```python
from build123d import *

# Parameters (mm, degrees)
SKETCH_1_W          = 32
SKETCH_1_H          = 86
EXTRUDE_1_DEPTH     = 3
SKETCH_2_W          = 12
SKETCH_2_H          = 3
SKETCH_2_W_2        = 3
CUT_EXTRUDE_1_DEPTH = 4
SKETCH_3_W          = 3
SKETCH_3_H          = 10
CUT_EXTRUDE_2_DEPTH = 4


with BuildPart() as part:
    # 스케치1 → 보스-돌출1 (new body)
    with BuildSketch(Plane.XY):
        with Locations((16, 43)):
            Rectangle(SKETCH_1_W, SKETCH_1_H)
    extrude(amount=EXTRUDE_1_DEPTH)

    # 스케치2 → 컷-돌출1 (cut, through all)
    with BuildSketch(Plane.XY.offset(3)):
        with Locations((16, 84.5)):
            Rectangle(SKETCH_2_W, SKETCH_2_H)
        with Locations((1.5, 84.5)):
            Rectangle(SKETCH_2_W_2, SKETCH_2_H)
        with Locations((30.5, 84.5)):
            Rectangle(SKETCH_2_W_2, SKETCH_2_H)
        with Locations((16, 1.5)):
            Rectangle(SKETCH_2_W, SKETCH_2_H)
        with Locations((1.5, 1.5)):
            Rectangle(SKETCH_2_W_2, SKETCH_2_H)
        with Locations((30.5, 1.5)):
            Rectangle(SKETCH_2_W_2, SKETCH_2_H)
    extrude(amount=-CUT_EXTRUDE_1_DEPTH, mode=Mode.SUBTRACT)

    # 스케치3 → 컷-돌출2 (cut, through all)
    with BuildSketch(Plane.XY.offset(3)):
        with Locations((27.5, 69)):
            Rectangle(SKETCH_3_W, SKETCH_3_H)
        with Locations((4.5, 69)):
            Rectangle(SKETCH_3_W, SKETCH_3_H)
        with Locations((27.5, 17)):
            Rectangle(SKETCH_3_W, SKETCH_3_H)
        with Locations((4.5, 17)):
            Rectangle(SKETCH_3_W, SKETCH_3_H)
    extrude(amount=-CUT_EXTRUDE_2_DEPTH, mode=Mode.SUBTRACT)


solid = part.part
```
Here's how the part is built. I have some questions about the finished solid (model axes, mm). A direction names the side the tool comes from. Give positions to 0.01 mm unless a question says otherwise; leave off trailing zeros. Loops run counter-clockwise (first coordinate to the right, second up) from the corner with the lowest first, then second, coordinate; pieces in that order, holes last. Notation, with made-up numbers: M 70,-10 L 122,-10 A23 ccw 122,10 Z; hole C 11.5,50.25 d4. An arc over 180 degrees is marked long. Put each result on its own line as item: value. Start each with the question number.
(1) I want a section at A-A on x = 4.5. Please give me the cut outline in (y, z).
(2) I want a section at B-B on y = 67.5. Please give me the cut outline in (x, z).
(3) If we mould it in two halves opening along X, with no side actions, what happens to faces 5 (the flat face through (3, 84, 2)), 6 (the flat face through (6, 0, 1)), 7 (the flat face through (22, 1, 2))? For each: +X half, -X half, draft (parallel to the pull), parting line (faces both ways), or undercut.
(4) I need wall thicknesses on line 1 along X through (y, z) = (66.5, 1.2); line 2 along Y through (x, z) = (28.5, 1.5); line 3 along Y through (x, z) = (17, 2.85). Which ranges of each line are inside material? Lowest first, please. Write a range as [from, to].
(5) I want a section at C-C on x = 13.5. Please give me the cut outline in (y, z).
(6) Will this pin go through, and if not, where does the flat tip stop? pin 1 Ø0.9 at (y, z) = (1, 1.5) entering from -X.
(7) For faces 1 (the flat face through (29, 84, 2)), 2 (the flat face through (3, 69, 2)), 3 (the flat face through (16, 83, 2)), 4 (the flat face through (1, 3, 2)), which set-ups out of +Z, -Z, +X, -X, +Y, -Y let a thin tool reach every point of the face, with its end or its side?
(8) I want a section at D-D on z = 0.7. State how many separate pieces and enclosed holes the cut face has, then the cut area to 3 significant figures.
Answer block:
1. outline: M 0,0 L 12,0 L 12,3 L 0,3 Z; M 22,0 L 64,0 L 64,3 L 22,3 Z; M 74,0 L 86,0 L 86,3 L 74,3 Z
2. outline: M 0,0 L 3,0 L 3,3 L 0,3 Z; M 6,0 L 26,0 L 26,3 L 6,3 Z; M 29,0 L 32,0 L 32,3 L 29,3 Z
3. face 5: -X half
3. face 6: draft
3. face 7: undercut
4. line 1: [0, 3], [6, 26], [29, 32]
4. line 2: [0, 12], [22, 64], [74, 86]
4. line 3: [3, 83]
5. outline: M 3,0 L 83,0 L 83,3 L 3,3 Z
6. pin 1: x = 3
7. face 1: +Z, -Z, +X, +Y
7. face 2: +Z, -Z
7. face 3: +Z, -Z, +Y
7. face 4: +Z, -Z, -X, -Y
8. separate pieces: 1
8. enclosed holes: 4
8. area: 2,520 mm^2
